Autodesk Inventor part; units mm, degrees
ref_plane "YZ Plane" through (0, 0, 0) normal (1, 0, 0) x (0, 1, 0)
ref_plane "XZ Plane" through (0, 0, 0) normal (0, 1, 0) x (-1, 0, 0)
ref_plane "XY Plane" through (0, 0, 0) normal (0, 0, 1) x (1, 0, 0)
sketch "Szkic1" plane through (0, 0, 0) normal (0, 0, 1) x (1, 0, 0)
  line L0 (-11.1928, -2.4042) -> (13.6072, -2.4042)
  line L1 (13.6072, -2.4042) -> (13.6072, 16.5958)
  line L2 (13.6072, 16.5958) -> (10.6072, 16.5958)
  line L3 (10.6072, 16.5958) -> (10.6072, 0.5958)
  line L4 (10.6072, 0.5958) -> (-11.1928, 0.5958)
  line L5 (-11.1928, 0.5958) -> (-11.1928, -2.4042)
  point P0 (0, 0)
  dimension "d0" = 24.8
  dimension "d1" = 19
  dimension "d2" = 3
  dimension "d3" = 16
extrude "Wyciągnięcie proste1" add sketch "Szkic1" along normal blind 20
fillet "Zaokrąglenie1" radius 5 2 edges at (-11.1928, -0.9042, 20) (-11.1928, -0.9042, 0)
fillet "Zaokrąglenie2" radius 3 1 edges at (10.6072, 0.5958, 10)
sketch "Szkic2" plane through (-11.1928, 0.5958, 15) normal (0, 1, 0) x (1, 0, 0)
  line L0 (18.8, 15) -> (18.8, -5)
  line L1 (18.8, 15) -> (5, 15)
  arc A0 (5, 15) -> (0, 10) centre (5, 10) ccw
  line L2 (0, 10) -> (0, 0)
  arc A1 (0, 0) -> (5, -5) centre (5, 0) ccw
  line L3 (18.8, -5) -> (5, -5)
  point P0 (11.1928, 15)
  point P1 (9.4, 5)
  dimension "d8" = 10
  dimension "d9" = 18.8
  dimension "d10" = 9.4
hole "Otwór1" at (-1.7928, 0.5958, 10) direction (0, -1, 0) diameter 5 depth 8 tip angle 118
sketch "Szkic3" plane through (10.6072, 16.5958, 0) normal (-1, 0, 0) x (0, 0, 1)
  line L0 (20, -13) -> (0, -13)
  line L1 (20, 0) -> (20, -13)
  line L2 (0, 0) -> (20, 0)
  line L3 (0, 0) -> (0, -13)
  point P0 (0, -16.5958)
  point P1 (6, -6)
  point P2 (14, -6)
  dimension "d18" = 6
  dimension "d19" = 6
  dimension "d20" = 6
  dimension "d21" = 6
hole "Otwór2" at (10.6072, 10.5958, 6) at (10.6072, 10.5958, 14) direction (1, 0, 0) diameter 3 depth 8 tip angle 118
properties part number "CNCM_ALU_3mm_Y_Axis_Idler_Stiffener_Side"
The listing builds one solid part. Answer for the finished solid, in the listing's coordinates (mm). A direction names the side the tool comes from. Round coordinates to 2 decimals unless told otherwise and drop trailing zeros. Loops run counter-clockwise (first coordinate to the right, second up) from the corner with the lowest first, then second, coordinate; pieces in that order, holes last. Notation, with made-up numbers: M 37,59.25 L 95,59.25 A17 ccw 95,88.25 Z; hole C 56,-21.75 d6. An arc over 180 degrees is marked long. Write each question's results on one line, items separated by ' | '. Start each with the question number.
1) Each of these flat-tipped pins is pushed along its axis until it touches: pin 1 (4 mm diameter, centred on x = -1.79, z = 10, fed in from -Y); pin 2 (10.5 mm diameter, centred on y = 11, z = 10.5, fed in from -X). Where does it stop, or does it pass through?
2) Which of the six approach directions +Z, -Z, +X, -X, +Y, -Y give full straight-line access (tool end or side, diameter ignored) to faces 1 (the flat face through (10.607, 10, 10)), 2 (the flat face through (12, 16.596, 10))?
3) Find section C-C on y = 5. Write down the section's boundary in (x, z).
4) Find section B-B on z = 14. Write down the section's boundary in (x, y), plus the area to 3 significant figures.
5) Determine the mould class of faces 3 (the flat face through (7, 0, 20)), 4 (the cylindrical face through (12.128, 9.582, 4.894)), 5 (the flat face through (0, 0.596, 8)) for opening direction Z: pulls with the +Z half, pulls with the -Z half, needs draft (parallel to the pull), parting line crosses it, or undercut.
6) Find section A-A on z = 10. Write down the section's boundary in (x, y), plus the area to 3 significant figures.
7) Find section D-D on z = 1.75. Write down the section's boundary in (x, y).
8) Straight lines are drawn through the part: probe 1 along Y at (x, z) = (11.85, 6); probe 2 along X at (y, z) = (-0.55, 10); probe 3 along Y at (x, z) = (2.75, 14.5). For each, find the intervals that lie inside material, in ascending order.
Final values:
1) pin 1: through | pin 2: x = 10.61
2) face 1: +Z, -Z, -X, +Y | face 2: +Z, -Z, +X, -X, +Y
3) outline: M 10.61,0 L 13.61,0 L 13.61,20 L 10.61,20 Z
4) outline: M -11.19,-2.4 L 13.61,-2.4 L 13.61,9.1 L 10.61,9.1 L 10.61,3.6 A3 cw 7.61,0.6 L -11.19,0.6 Z; M 10.61,12.1 L 13.61,12.1 L 13.61,16.6 L 10.61,16.6 Z | area: 115 mm²
5) face 3: pulls with the +Z half | face 4: undercut | face 5: needs draft
6) outline: M -11.19,-2.4 L -4.29,-2.4 L -4.29,0.6 L -11.19,0.6 Z; M 0.71,-2.4 L 13.61,-2.4 L 13.61,16.6 L 10.61,16.6 L 10.61,3.6 A3 cw 7.61,0.6 L 0.71,0.6 Z | area: 109 mm²
7) outline: M -9.99,-2.4 L 13.61,-2.4 L 13.61,16.6 L 10.61,16.6 L 10.61,3.6 A3 cw 7.61,0.6 L -9.99,0.6 Z
8) probe 1: -2.4 to 9.1, 12.1 to 16.6 | probe 2: -11.19 to -4.29, 0.71 to 13.61 | probe 3: -2.4 to 0.6
